Here's how the part is built. I have some questions about the finished solid (model axes, mm). Face numbers are marked on the shaded views. A direction names the side the tool comes from. Round coordinates to 2 decimals unless told otherwise and drop trailing zeros. Order: outer loops, then holes, each group sorted by start corner. A loop starts at its lowest first (then second) coordinate and runs counter-clockwise, first axis right, second up. Notation, with made-up numbers: M 0,19 L 4,19 A26 cw 4,58 Z; hole C -15.75,20 d5. An arc over 180 degrees is marked long. Write item = value, one per line. Start each with the question number.
Item 1: For the marked faces 1 and 2, which set-ups out of +Z, -Z, +X, -X, +Y, -Y let a thin tool reach every point of the face, with its end or its side?
Item 2: I'm going to push flat-ended pins straight in: P1, Ø6, axis at y = 49.5, z = 7.5, coming from the -X side; P2, Ø8, axis at x = -5, y = 33.5, coming from the -Z side; P3, Ø12, axis at x = 4.5, y = 22, coming from the +Z side. Where does each tip first touch, or does it pass through?
Item 3: Please list where these lines run through material, in increasing order: L1, parallel to X at y = 16.15, z = 0; L2, parallel to Y at x = 0.5, z = -8.25; L3, parallel to Y at x = -4, z = -2.
Item 4: I want a section at B-B, the plane y = 45. List the corners of the cut face in (x, z) for me.
Item 5: I want a section at D-D, the plane y = 28. List the corners of the cut face in (x, z) for me, plus the area to 3 significant figures.
Item 6: I want a section at A-A, the plane z = 4.5. State how many separate pieces and enclosed holes the cut face has, plus the area to 3 significant figures.
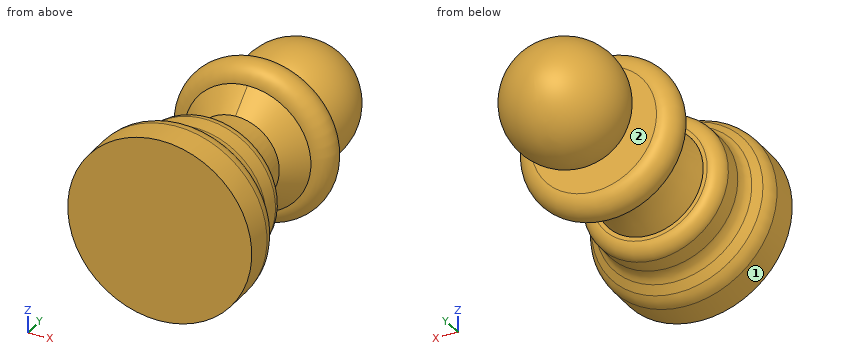
```python
from build123d import *

# Parameters (mm, degrees)
CUT_EXTRUDE1_START = -0.4
SKETCH4_R          = 10
CUT_EXTRUDE1_DEPTH = 2.56


with BuildPart() as part:
    # Sketch1 → Revolve1 (revolve)
    with BuildSketch(Plane.XY, mode=Mode.PRIVATE) as revolve1_sk:
        with BuildLine():
            Line((-11.6, 16.590020296), (-11.6, 17.708076526))
            ThreePointArc((-11.6, 17.708076526), (-11.393009972, 18.715730197), (-10.805562363, 19.560192215))
            Line((-10.805562363, 19.560192215), (-9.867833159, 20.452169234))
            ThreePointArc((-9.867833159, 20.452169234), (-9.28038555, 21.296631251), (-9.073395522, 22.304284923))
            Line((-9.073395522, 22.304284923), (-9.073395522, 24.568565429))
            ThreePointArc((-9.073395522, 24.568565429), (-8.5606623, 25.806412928), (-7.322814801, 26.31914615))
            Line((-7.322814801, 26.31914615), (-6.816009802, 26.31914615))
            ThreePointArc((-6.816009802, 26.31914615), (-5.724674741, 30.659629783), (-5.412117665, 35.124281892))
            Line((-5.412117665, 35.124281892), (-7.908297127, 35.124281892))
            ThreePointArc((-7.908297127, 35.124281892), (-10.158297127, 37.374281892), (-7.908297127, 39.624281892))
            Line((-7.908297127, 39.624281892), (-2.916866685, 39.624281892))
            ThreePointArc((-2.916866685, 39.624281892), (-7.350905696, 48.021846367), (0, 54.033832438))
            Line((0, 54.033832438), (0, 14.033832438))
            Line((0, 14.033832438), (-9.043812142, 14.033832438))
            Line((-9.043812142, 14.033832438), (-11.6, 14.033832438))
            Line((-11.6, 14.033832438), (-11.6, 16.590020296))
        make_face()
    revolve(revolve1_sk.sketch.rotate(Axis((0, -5.761492399, 0), (0, 1, 0)), 270), axis=Axis((0, -5.761492399, 0), (0, 1, 0)))

    # Chamfer1: read off the stored shape, not the designer's step
    # Chamfer1: loft between two sections, ruled curve by curve
    chamfer1_from = [
        Edge.make_three_point_arc((0, 32.247480775, 5.522579882), (5.522579882, 32.247480775, 0), (0, 32.247480775, -5.522579882)),
        Edge.make_three_point_arc((0, 32.247480775, -5.522579882), (-5.522579882, 32.247480775, 0), (0, 32.247480775, 5.522579882)),
    ]
    chamfer1_to = [
        Edge.make_three_point_arc((0, 35.125992507, 7.996017369), (7.996017369, 35.125992507, 0), (0, 35.125992507, -7.996017369)),
        Edge.make_three_point_arc((0, 35.125992507, -7.996017369), (-7.996017369, 35.125992507, 0), (0, 35.125992507, 7.996017369)),
    ]
    chamfer1 = Solid(Shell([*[Face.make_surface_from_curves(chamfer1_from[k], chamfer1_to[k]) for k in range(2)], Face(Wire(chamfer1_from)), Face(Wire(chamfer1_to))]))
    add(chamfer1)

    # Sketch4 → Cut-Extrude1 (cut)
    with BuildSketch(Plane.XZ.offset(-14.033832438).offset(CUT_EXTRUDE1_START)):
        with Locations(Location((0, 0, 0), (0, 0, 270))):
            Circle(SKETCH4_R)
    extrude(amount=-CUT_EXTRUDE1_DEPTH, mode=Mode.SUBTRACT)


solid = part.part
```
Filled in:
q1.face_1 = +Y, -Y
q1.face_2 = none
q2.P1 = -5.53
q2.P2 = -9.71
q2.P3 = 11.6
q3.L1 = -11.6 to -10, 10 to 11.6
q3.L2 = 14.03 to 14.43, 16.99 to 26.04, 35.15 to 39.6
q3.L3 = 14.03 to 14.43, 16.99 to 39.62, 40.51 to 52.55
q4.outline = C 0,0 d14.68
q5.outline = C 0,0 d12.59
q5.area = 125 mm^2
q6.separate_pieces = 2
q6.enclosed_holes = 1
q6.area = 447 mm^2
